Verification items for the finished model (mm, model axes). Coordinates: 2 decimals unless noted, no trailing zeros. Use a Markdown table: item, result. Add a question column.
Autodesk Inventor part; units mm, degrees
ref_plane "Work Plane1" through (1104.5696, 91.5553, 211.8164) normal (0, 1, 0) x (-1, 0, 0)
ref_plane "YZ Plane" through (0, 0, 0) normal (1, 0, 0) x (0, 1, 0)
ref_plane "XZ Plane" through (0, 0, 0) normal (0, 1, 0) x (-1, 0, 0)
ref_plane "Work Plane1" through (1104.5696, 91.5553, 211.8164) normal (0, 1, 0) x (-1, 0, 0)
sketch "Sketch1" plane through (1104.5696, 91.5553, 211.8164) normal (0, 1, 0) x (-1, 0, 0)
  arc A0 (57.6551, 1254.9955) -> (57.6551, 1150.0245) centre (104.395, 1202.51) ccw
  line L0 (-26.3951, 1291) -> (133.6049, 1291)
  line L1 (133.6049, 1019) -> (-26.3951, 1019)
  line L2 (-26.3951, 1249) -> (-26.3951, 1291)
  line L3 (179.6049, 2285) -> (179.6049, 25)
  line L4 (179.6049, 1019) -> (179.6049, 1291.0001)
  line L5 (-72.3951, 25) -> (-72.3951, 2285)
  line L6 (179.6049, 1291.0001) -> (-222.3951, 1291.0001)
  line L7 (179.6049, 1019) -> (-222.3951, 1019)
  line L8 (-222.3951, 25) -> (-222.3951, 2285)
  line L9 (-222.3951, 1291.0001) -> (-222.3951, 1019)
  point P0 (1104.5696, -211.8164)
  point P1 (-72.3951, 1291.0001)
  point P2 (-72.3951, 1019)
  point P3 (154, 1291)
  point P4 (4, 1291)
extrude "Extrusion1" add sketch "Sketch1" along normal blind 12.7
sketch "Sketch2" plane through (1104.5696, 104.2553, 211.8164) normal (0, 1, 0) x (1, 0, 0)
  line L0 (222.3951, -1019) -> (-179.6049, -1019) construction
  line L1 (-179.6049, -1019) -> (-179.6049, -1291.0001) construction
  line L2 (-179.6049, -1291.0001) -> (222.3951, -1291.0001) construction
  line L3 (222.3951, -1291.0001) -> (222.3951, -1019) construction
  line L4 (-179.6049, -1291.0001) -> (222.3951, -1291.0001) construction
  line L5 (21.3951, -1291.0001) -> (21.3951, -1019) construction
  line L6 (-179.6049, -1019) -> (-179.6049, -1291.0001) construction
  line L7 (-179.6049, -1155) -> (222.3951, -1155) construction
  point P0 (-1104.5696, 211.8164)
  point P1 (-159.6049, -1266.0001)
  point P2 (165.3951, -1266.0001)
  point P3 (-159.6049, -1044)
  point P4 (165.3951, -1044)
  dimension "d16" = 25
  dimension "d17" = 20
  dimension "d18" = 25
  dimension "d19" = 325
hole "Hole1" at (944.9647, 104.2553, 1477.8164) at (944.9647, 104.2553, 1255.8164) at (1269.9647, 104.2553, 1255.8164) at (1269.9647, 104.2553, 1477.8164) direction (0, -1, 0) diameter 12 end through all
sketch "Sketch3" plane through (1104.5696, 104.2553, 211.8164) normal (0, 1, 0) x (1, 0, 0)
  line L0 (-129.6049, -1110.5) -> (-40.6049, -1110.5)
  line L1 (-40.6049, -1110.5) -> (-40.6049, -1199.5)
  line L2 (-40.6049, -1199.5) -> (-129.6049, -1199.5)
  line L3 (-129.6049, -1199.5) -> (-129.6049, -1110.5)
  line L4 (-179.6049, -1019) -> (-179.6049, -1291.0001)
  line L5 (-179.6049, -1155) -> (-143.519, -1155)
  point P0 (-1104.5696, 211.8164)
  dimension "d20" = 89
  dimension "d21" = 89
  dimension "d22" = 50
hole "Hole2" at (974.9647, 104.2553, 1322.3164) at (1063.9647, 104.2553, 1322.3164) at (1063.9647, 104.2553, 1411.3164) at (974.9647, 104.2553, 1411.3164) direction (0, -1, 0) diameter 10 end through all
properties part number "PlacaInferior" material "Steel ASTM A36"
1) Thickness scan on L1, parallel to Z at x = 1266, y = 93.75; L2, parallel to X at y = 96, z = 1473. Record the ranges inside material, lowest first.
2) Gauge pin test, flat ends, axial feed: pin 1 (19 mm diameter, centred on x = 944.96, z = 1477.82, fed in from -Y); pin 2 (6 mm diameter, centred on x = 1063.96, z = 1322.32, fed in from -Y). Record the tip position at first contact, or that the pin passes through.
3) Release check for a two-part mould opening along Z. For faces 1 (the face through (1123, 98, 1230.816)), 2 (the face through (970.007, 97.816, 1321.665)), 3 (the face through (1129, 91.555, 1369)) record: released by +Z, released by -Z, zero draft, split by the parting line, or undercut.
Returned:
| question | item | result |
|---|---|---|
| 1 | L1 | z = 1230.82 to 1251.31, 1260.32 to 1473.31, 1482.32 to 1502.82 |
| 1 | L2 | x = 924.96 to 941.39, 948.54 to 1266.39, 1273.54 to 1326.96 |
| 2 | pin 1 | stops at y = 91.56 |
| 2 | pin 2 | passes through |
| 3 | face 1 | released by -Z |
| 3 | face 2 | undercut |
| 3 | face 3 | zero draft |
